```python
from build123d import *

# Parameters (mm, degrees)
SKETCH_1_R      = 1.5
EXTRUDE_1_DEPTH = 1
SKETCH_2_W      = 5
SKETCH_2_H      = 22
EXTRUDE_2_DEPTH = 1
EXTRUDE_START   = 21
SKETCH_1_2_R    = 1.5
EXTRUDE_3_DEPTH = 1
EXTRUDE_START_2 = 11
SKETCH_1_3_R    = 1.5
EXTRUDE_4_DEPTH = 0.5
SKETCH_3_R      = 2.5
EXTRUDE_5_DEPTH = 4
EXTRUDE_6_REACH = 39.766
EXTRUDE_7_REACH = 39.766
SKETCH_5_R      = 4.5
SKETCH_5_R_2    = 1.5


with BuildPart() as part:
    # 草图1 → 凸台-拉伸1 (new body)
    with BuildSketch(Plane.XY):
        with BuildLine():
            Line((-2.5, 26), (-6.421436, 1.007554))
            ThreePointArc((-6.421436, 1.007554), (0, -6.5), (6.421436, 1.007554))
            Line((6.421436, 1.007554), (2.5, 26))
            Line((2.5, 26), (-2.5, 26))
        make_face()
        Circle(SKETCH_1_R, mode=Mode.SUBTRACT)
    extrude(amount=EXTRUDE_1_DEPTH)

    # 草图2 → 凸台-拉伸2 (add)
    with BuildSketch(Plane(origin=(0, 26, 0), x_dir=(1, 0, 0), z_dir=(0, 1, 0))):
        with Locations((0, -11)):
            Rectangle(SKETCH_2_W, SKETCH_2_H)
    extrude(amount=-EXTRUDE_2_DEPTH)

    # 草图1<2> → 凸台-拉伸3 (add)
    with BuildSketch(Plane.XY.offset(EXTRUDE_START)):
        with BuildLine():
            Line((-2.5, 26), (-6.421436, 1.007554))
            ThreePointArc((-6.421436, 1.007554), (0, -6.5), (6.421436, 1.007554))
            Line((6.421436, 1.007554), (2.5, 26))
            Line((2.5, 26), (-2.5, 26))
        make_face()
        Circle(SKETCH_1_2_R, mode=Mode.SUBTRACT)
    extrude(amount=EXTRUDE_3_DEPTH)

    # 草图1<3> → 凸台-拉伸4 (add, symmetric)
    with BuildSketch(Plane.XY.offset(EXTRUDE_START_2)):
        with BuildLine():
            Line((-2.5, 26), (-6.421436, 1.007554))
            ThreePointArc((-6.421436, 1.007554), (0, -6.5), (6.421436, 1.007554))
            Line((6.421436, 1.007554), (2.5, 26))
            Line((2.5, 26), (-2.5, 26))
        make_face()
        Circle(SKETCH_1_3_R, mode=Mode.SUBTRACT)
    extrude(amount=EXTRUDE_4_DEPTH, both=True)

    # 草图3 → 凸台-拉伸5 (add)
    with BuildSketch(Plane(origin=(0, 26, 0), x_dir=(1, 0, 0), z_dir=(0, 1, 0))):
        with Locations(Location((0, -11, 0), (0, 0, 180))):
            Circle(SKETCH_3_R)
    extrude(amount=EXTRUDE_5_DEPTH)

    # 凸台-拉伸6: up to this face of the body (flat: up to its plane)
    extrude_6_end = Plane(part.part.faces().sort_by_distance((0, 8.21558, 22))[0])
    # 草图4 → 凸台-拉伸6 (add, up to the picked face)
    with BuildSketch(Plane(origin=(0, 0, 0), x_dir=(-1, 0, 0), z_dir=(0, 0, -1)), mode=Mode.PRIVATE) as extrude_6_sk1:
        with BuildLine():
            Line((-2.75, -4.76314), (-3.25, -5.629165))
            ThreePointArc((-3.25, -5.629165), (0, -6.5), (3.25, -5.629165))
            Line((3.25, -5.629165), (2.75, -4.76314))
            ThreePointArc((2.75, -4.76314), (0, -5.5), (-2.75, -4.76314))
        make_face()
    extrude_6_tool1 = split(extrude(extrude_6_sk1.sketch, amount=-EXTRUDE_6_REACH, mode=Mode.PRIVATE), bisect_by=extrude_6_end, keep=Keep.BOTH, mode=Mode.PRIVATE)
    add(extrude_6_tool1.solids().sort_by(Axis((0, -5.742841, 0), (0, 0, 1)))[0])

    # 凸台-拉伸7: up to this face of the body (flat: up to its plane)
    extrude_7_end = Plane(part.part.faces().sort_by_distance((0, 8.21558, 22))[0])
    # 草图5 → 凸台-拉伸7 (add, up to the picked face)
    with BuildSketch(Plane(origin=(0, 0, 0), x_dir=(-1, 0, 0), z_dir=(0, 0, -1)), mode=Mode.PRIVATE) as extrude_7_sk1:
        with Locations(Location((0, 0, 0), (0, 0, 180))):
            Circle(SKETCH_5_R)
        with Locations(Location((0, 0, 0), (0, 0, 180))):
            Circle(SKETCH_5_R_2, mode=Mode.SUBTRACT)
    extrude_7_tool1 = split(extrude(extrude_7_sk1.sketch, amount=-EXTRUDE_7_REACH, mode=Mode.PRIVATE), bisect_by=extrude_7_end, keep=Keep.BOTH, mode=Mode.PRIVATE)
    add(extrude_7_tool1.solids().sort_by(Axis((-4.372721, 0, 0), (0, 0, 1)))[0])


solid = part.part
```
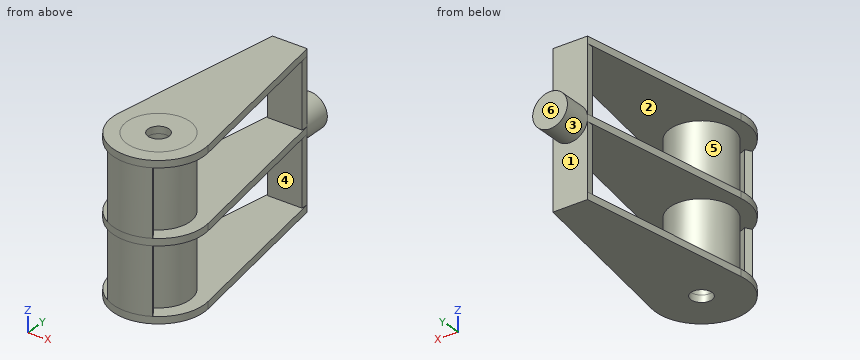
The listing builds one solid part. Answer for the finished solid, in the listing's coordinates (mm). Face numbers are marked on the shaded views. A direction names the side the tool comes from. Give positions to 0.01 mm unless a question says otherwise; leave off trailing zeros. Order: outer loops, then holes, each group sorted by start corner. A loop starts at its lowest first (then second) coordinate and runs counter-clockwise, first axis right, second up.
1) Consider line 1 along Z through (x, y) = (-1.5, 11); line 2 along Y through (x, z) = (0, 17.75); line 3 along Y through (x, z) = (1.75, 10.25). Determine where each line is inside the solid, lowest interval first.
Reported:
line 1: z = 0 to 1, 10.5 to 11.5, 21 to 22
line 2: y = -6.5 to -5.5, -4.5 to -1.5, 1.5 to 4.5, 25 to 26
line 3: y = -6.26 to -5.21, -4.15 to 4.15, 25 to 30
2) Determine the mould class of the marked faces 1, 2 and 3 for opening direction Y: pulls with the +Y half, pulls with the -Y half, needs draft (parallel to the pull), parting line crosses it, or undercut.
Reported:
face 1: pulls with the +Y half
face 2: undercut
face 3: needs draft
3) Find section A-A on x = 0. Write down the section's boundary in (y, z), then the cut area to 4 significant figures.
Reported:
outline: (-6.5, 0) - (-1.5, 0) - (-1.5, 22) - (-6.5, 22) - close; (1.5, 0) - (26, 0) - (26, 8.5) - (30, 8.5) - (30, 13.5) - (26, 13.5) - (26, 22) - (1.5, 22) - close; hole (-5.5, 1) - (-4.5, 1) - (-4.5, 10.5) - (-5.5, 10.5) - close; hole (-5.5, 11.5) - (-4.5, 11.5) - (-4.5, 21) - (-5.5, 21) - close; hole (4.5, 1) - (25, 1) - (25, 10.5) - (4.5, 10.5) - close; hole (4.5, 11.5) - (25, 11.5) - (25, 21) - (4.5, 21) - close
area: 260.5 mm2
4) Find section D-D on y = 12.5. Write down the section's boundary in (x, z).
Reported:
outline: (-4.62, 0) - (4.62, 0) - (4.62, 1) - (-4.62, 1) - close; (-4.62, 10.5) - (4.62, 10.5) - (4.62, 11.5) - (-4.62, 11.5) - close; (-4.62, 21) - (4.62, 21) - (4.62, 22) - (-4.62, 22) - close
5) Find section C-C on y = 0. Write down the section's boundary in (x, z).
Reported:
outline: (-6.5, 0) - (-1.5, 0) - (-1.5, 22) - (-6.5, 22) - (-6.5, 21) - (-4.5, 21) - (-4.5, 11.5) - (-6.5, 11.5) - (-6.5, 10.5) - (-4.5, 10.5) - (-4.5, 1) - (-6.5, 1) - close; (1.5, 0) - (6.5, 0) - (6.5, 1) - (4.5, 1) - (4.5, 10.5) - (6.5, 10.5) - (6.5, 11.5) - (4.5, 11.5) - (4.5, 21) - (6.5, 21) - (6.5, 22) - (1.5, 22) - close
6) For the marked faces 4, 5 and 6, determine the directions among +Z, -Z, +X, -X, +Y, -Y from which every point of the face is accessible in a straight line to the end or side of a thin tool.
Reported:
face 4: +X, -X
face 5: none
face 6: +Z, -Z, +X, -X, +Y
7) Given P1, Ø0.5, axis at y = 25.5, z = 5.5, coming from the -X side; P2, Ø3.5, axis at x = 0, y = 0, coming from the -Z side; P3, Ø6, axis at y = 17, z = 3, coming from the -X side; P4, Ø5, axis at y = 5.5, z = 12.5, coming from the +X side, each flat-ended and moving along its own axis, determine where each tip first touches the part or whether it passes through.
Reported:
P1: stops at x = -2.5
P2: stops at z = 0
P3: stops at x = -4.26
P4: stops at x = 6.08
8) Find section B-B on z = 4. Write down the section's boundary in (x, y).
Reported:
outline: circle Ø9 at (0, 0); (-3.25, -5.63) arc R6.5 ccw to (3.25, -5.63) - (2.75, -4.76) arc R5.5 cw to (-2.75, -4.76) - close; (-2.5, 25) - (2.5, 25) - (2.5, 26) - (-2.5, 26) - close; hole circle Ø3 at (0, 0)
